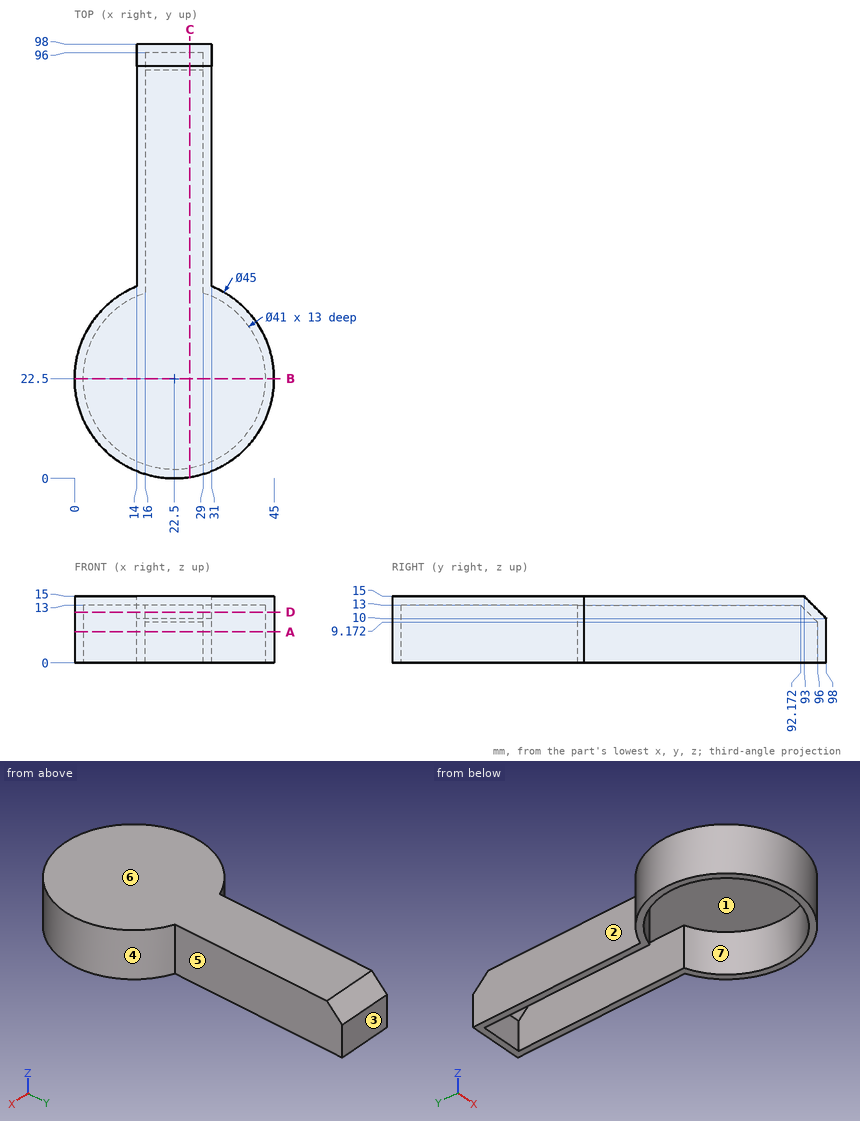
Verification items for this drawing (mm, ordinates from the low corner). A direction names the side the tool comes from. Give positions to 0.01 mm unless a question says otherwise; leave off trailing zeros. Loops run counter-clockwise (first coordinate to the right, second up) from the corner with the lowest first, then second, coordinate; pieces in that order, holes last. Notation, with made-up numbers: M 16,1.5 L 56,1.5 A26 ccw 56,19.5 Z; hole C 74.5,-21 d10. An arc over 180 degrees is marked long. Answer in a Markdown table with one row per item.
1) Mould release check, pull along X, two halves, no side actions. Record for the marked faces 4, 5, 6 and 7: released by +X, released by -X, zero draft, split by the parting line, or undercut.
Solutions:
| item | result |
|---|---|
| face 4 | split by the parting line |
| face 5 | released by +X |
| face 6 | zero draft |
| face 7 | undercut |
2) Cross-section at D-D (z = 11.5). Enter the section's corners in (x, y).
Solutions:
| item | result |
|---|---|
| outline | M 14,43.33 A22.5 ccw long 31,43.33 L 31,96.5 L 14,96.5 Z; hole M 16,41.94 A20.5 ccw long 29,41.94 L 29,93.67 L 16,93.67 Z |
3) Thickness scan on line 1 (X direction, y = 22.5, z = 8.25); line 2 (Y direction, x = 22.5, z = 7.25); line 3 (X direction, y = 54.5, z = 10.25). Record the ranges inside material, lowest first.
Solutions:
| item | result |
|---|---|
| line 1 | x = 0 to 2, 43 to 45 |
| line 2 | y = 0 to 2, 96 to 98 |
| line 3 | x = 14 to 16, 29 to 31 |
4) Depth check by flat-ended pin: pin 1 (5 mm diameter, centred on y = 29, z = 6.5, fed in from +X); pin 2 (24.5 mm diameter, centred on x = 22.5, y = 22.5, fed in from -Z); pin 3 (4 mm diameter, centred on y = 29.5, z = 4, fed in from -X); pin 4 (3 mm diameter, centred on x = 23.5, z = 6.5, fed in from -Y). Enter the tip coordinate at first touch or a pass-through.
Solutions:
| item | result |
|---|---|
| pin 1 | stops at x = 44.64 |
| pin 2 | stops at z = 13 |
| pin 3 | stops at x = 0.56 |
| pin 4 | stops at y = 0 |
5) Cross-section at B-B (y = 22.5). Enter the section's corners in (x, z).
Solutions:
| item | result |
|---|---|
| outline | M 0,0 L 2,0 L 2,13 L 43,13 L 43,0 L 45,0 L 45,15 L 0,15 Z |
6) Cross-section at A-A (z = 7). Enter the section's corners in (x, y).
Solutions:
| item | result |
|---|---|
| outline | M 14,43.33 A22.5 ccw long 31,43.33 L 31,98 L 14,98 Z; hole M 16,41.94 A20.5 ccw long 29,41.94 L 29,96 L 16,96 Z |
7) Cross-section at C-C (x = 26). Enter the section's corners in (y, z).
Solutions:
| item | result |
|---|---|
| outline | M 0.27,0 L 2.3,0 L 2.3,13 L 92.17,13 L 96,9.17 L 96,0 L 98,0 L 98,10 L 93,15 L 0.27,15 Z |
8) Tool access check on the marked faces 1, 2 and 3. Record the directions out of +Z, -Z, +X, -X, +Y, -Y that give a thin tool (end or side, any length) a straight path to the whole face; none if there is none.
Solutions:
| item | result |
|---|---|
| face 1 | -Z |
| face 2 | +Z, -Z, -X, +Y |
| face 3 | +Z, -Z, +X, -X, +Y |
